from build123d import *

# Parameters (mm, degrees)
SKETCH1_R           = 2.5019
BOSS_EXTRUDE1_DEPTH = 110.9472
SKETCH2_R           = 19.05
BOSS_EXTRUDE2_DEPTH = 1.5875
SKETCH3_R           = 4.0005
BOSS_EXTRUDE3_DEPTH = 20.5994
CUT_EXTRUDE1_DEPTH  = 105.791


with BuildPart() as part:
    # Sketch1 → Boss-Extrude1 (new body)
    with BuildSketch(Plane.XY):
        with BuildLine():
            Line((-34.002396427, 28.194), (18.143803573, 28.194))
            ThreePointArc((18.143803573, 28.194), (19.643506345, 27.572802772), (20.264703573, 26.0731))
            Line((20.264703573, 26.0731), (20.264703573, -26.0731))
            ThreePointArc((20.264703573, -26.0731), (19.643506345, -27.572802772), (18.143803573, -28.194))
            Line((18.143803573, -28.194), (-34.002396427, -28.194))
            ThreePointArc((-34.002396427, -28.194), (-35.502099199, -27.572802772), (-36.123296427, -26.0731))
            Line((-36.123296427, -26.0731), (-36.123296427, 26.0731))
            ThreePointArc((-36.123296427, 26.0731), (-35.502099199, 27.572802772), (-34.002396427, 28.194))
        make_face()
        with Locations((15.641903573, 23.5712)):
            Circle(SKETCH1_R, mode=Mode.SUBTRACT)
        with Locations(Location((-31.500496427, 23.5712, 0), (0, 0, 180))):
            Circle(SKETCH1_R, mode=Mode.SUBTRACT)
        with Locations((-31.500496427, -23.5712)):
            Circle(SKETCH1_R, mode=Mode.SUBTRACT)
        with Locations(Location((15.641903573, -23.5712, 0), (0, 0, 180))):
            Circle(SKETCH1_R, mode=Mode.SUBTRACT)
    extrude(amount=BOSS_EXTRUDE1_DEPTH)

    # Sketch2 → Boss-Extrude2 (add)
    with BuildSketch(Plane.XY.offset(110.9472)):
        with Locations((-7.929296427, 0)):
            Circle(SKETCH2_R)
    extrude(amount=BOSS_EXTRUDE2_DEPTH)

    # Sketch3 → Boss-Extrude3 (add)
    with BuildSketch(Plane.XY.offset(112.5347)):
        with Locations((-7.929296427, 0)):
            Circle(SKETCH3_R)
    extrude(amount=BOSS_EXTRUDE3_DEPTH)

    # Sketch4 → Cut-Extrude1 (cut)
    with BuildSketch(Plane(origin=(0, 0, 0), x_dir=(-1, 0, 0), z_dir=(0, 0, -1))):
        with BuildLine():
            Line((34.535796427, -19.177), (33.456296427, -19.177))
            ThreePointArc((33.456296427, -19.177), (28.966168367, -21.036871939), (27.106296427, -25.527))
            Line((27.106296427, -25.527), (27.106296427, -26.6065))
            ThreePointArc((27.106296427, -26.6065), (26.641328442, -27.729032015), (25.518796427, -28.194))
            Line((25.518796427, -28.194), (18.677208221, -28.194))
            Line((18.677208221, -28.194), (18.677208221, -39.079996732))
            Line((18.677208221, -39.079996732), (53.323924266, -39.079996732))
            Line((53.323924266, -39.079996732), (53.323924266, -7.667262783))
            Line((53.323924266, -7.667262783), (36.123296427, -7.667262783))
            Line((36.123296427, -7.667262783), (36.123296427, -17.5895))
            ThreePointArc((36.123296427, -17.5895), (35.658328442, -18.712032015), (34.535796427, -19.177))
        make_face()
        with BuildLine():
            Line((36.123296427, 7.667262783), (36.123296427, 17.5895))
            ThreePointArc((36.123296427, 17.5895), (35.658328442, 18.712032015), (34.535796427, 19.177))
            Line((34.535796427, 19.177), (33.456296427, 19.177))
            ThreePointArc((33.456296427, 19.177), (28.966168367, 21.036871939), (27.106296427, 25.527))
            Line((27.106296427, 25.527), (27.106296427, 26.6065))
            ThreePointArc((27.106296427, 26.6065), (26.641328442, 27.729032015), (25.518796427, 28.194))
            Line((25.518796427, 28.194), (18.677208221, 28.194))
            Line((18.677208221, 28.194), (18.677208221, 39.079996732))
            Line((18.677208221, 39.079996732), (53.323924266, 39.079996732))
            Line((53.323924266, 39.079996732), (53.323924266, 7.667262783))
            Line((53.323924266, 7.667262783), (36.123296427, 7.667262783))
        make_face()
        with BuildLine():
            Line((-18.677203573, 19.177), (-17.597703573, 19.177))
            ThreePointArc((-17.597703573, 19.177), (-13.107575512, 21.036871939), (-11.247703573, 25.527))
            Line((-11.247703573, 25.527), (-11.247703573, 26.6065))
            ThreePointArc((-11.247703573, 26.6065), (-10.782735588, 27.729032015), (-9.660203573, 28.194))
            Line((-9.660203573, 28.194), (-2.818615366, 28.194))
            Line((-2.818615366, 28.194), (-2.818615366, 39.079996732))
            Line((-2.818615366, 39.079996732), (-37.465331412, 39.079996732))
            Line((-37.465331412, 39.079996732), (-37.465331412, 7.667262783))
            Line((-37.465331412, 7.667262783), (-20.264703573, 7.667262783))
            Line((-20.264703573, 7.667262783), (-20.264703573, 17.5895))
            ThreePointArc((-20.264703573, 17.5895), (-19.799735588, 18.712032015), (-18.677203573, 19.177))
        make_face()
        with BuildLine():
            Line((-20.264703573, -7.667262783), (-20.264703573, -17.5895))
            ThreePointArc((-20.264703573, -17.5895), (-19.799735588, -18.712032015), (-18.677203573, -19.177))
            Line((-18.677203573, -19.177), (-17.597703573, -19.177))
            ThreePointArc((-17.597703573, -19.177), (-13.107575512, -21.036871939), (-11.247703573, -25.527))
            Line((-11.247703573, -25.527), (-11.247703573, -26.6065))
            ThreePointArc((-11.247703573, -26.6065), (-10.782735588, -27.729032015), (-9.660203573, -28.194))
            Line((-9.660203573, -28.194), (-2.818615366, -28.194))
            Line((-2.818615366, -28.194), (-2.818615366, -39.079996732))
            Line((-2.818615366, -39.079996732), (-37.465331412, -39.079996732))
            Line((-37.465331412, -39.079996732), (-37.465331412, -7.667262783))
            Line((-37.465331412, -7.667262783), (-20.264703573, -7.667262783))
        make_face()
    extrude(amount=-CUT_EXTRUDE1_DEPTH, mode=Mode.SUBTRACT)


solid = part.part
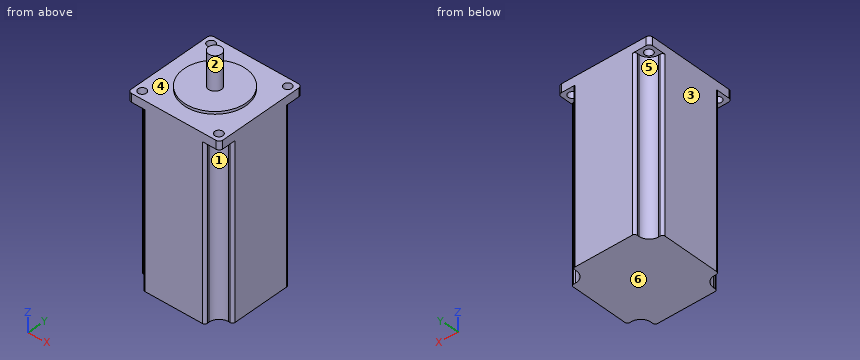
Here's how the part is built. I have some questions about the finished solid (model axes, mm). Face numbers are marked on the shaded views. A direction names the side the tool comes from. Coordinates: 2 decimals unless noted, no trailing zeros. Write each loop counter-clockwise with the first axis right and the second up, starting at its lowest first coordinate (ties: lowest second). Pieces come first, ordered by that corner, then holes. Notation, with made-up numbers: (28, 20.5) - (42, 20.5) arc R17 ccw to (42, 27.5) - close; hole circle Ø11 at (87.25, -10.75). An arc over 180 degrees is marked (long way). Use one line per item in the form item = value.
1) I need wall thicknesses on line 1 (Z direction, x = 12, y = 2.5); line 2 (Z direction, x = -12, y = -16.5); line 3 (X direction, y = -25, z = 6). Which ranges of each line are inside material? Lowest first, please.
Solved:
line_1 = 0 to 110.95
line_2 = 0 to 112.53
line_3 = -27.13 to 11.27
2) Suppose I cut it at D-D, the plane x = -19.5. Write out the boundary of the cut face in (y, z).
Solved:
outline = (-28.19, 0) - (28.19, 0) - (28.19, 110.95) - (15.13, 110.95) - (15.13, 112.53) - (-15.13, 112.53) - (-15.13, 110.95) - (-28.19, 110.95) - close
3) Suppose I cut it at B-B, the plane x = -31.5. Write out the boundary of the cut face in (y, z).
Solved:
outline = (-28.19, 105.79) - (-26.07, 105.79) - (-26.07, 110.95) - (-28.19, 110.95) - close; (-21.07, 105.79) - (-19.49, 105.79) - (-19.49, 0) - (19.49, 0) - (19.49, 105.79) - (21.07, 105.79) - (21.07, 110.95) - (-21.07, 110.95) - close; (26.07, 105.79) - (28.19, 105.79) - (28.19, 110.95) - (26.07, 110.95) - close
4) Suppose I cut it at A-A, the plane y = 0. Write out the boundary of the cut face in (x, z).
Solved:
outline = (-36.12, 0) - (20.26, 0) - (20.26, 110.95) - (11.12, 110.95) - (11.12, 112.53) - (-3.93, 112.53) - (-3.93, 133.13) - (-11.93, 133.13) - (-11.93, 112.53) - (-26.98, 112.53) - (-26.98, 110.95) - (-36.12, 110.95) - close
5) I'm going to push flat-ended pins straight in: P1, Ø1, axis at x = 7.5, y = -22, coming from the +Z side; P2, Ø0.9, axis at y = 26, z = 54, coming from the -X side; P3, Ø1.2, axis at y = -26, z = 76, coming from the +X side. Where does each tip first touch, or does it pass through?
Solved:
P1 = 110.95
P2 = -27.11
P3 = 11.25
6) On a 3-axis mill with a long thin cutter (end or side, diameter ignored), from which of +Z, -Z, +X, -X, +Y, -Y can I reach the whole of each face in a straight line? I mean the marked faces 1, 2 and 3. Say none if no direction works.
Solved:
face_1 = -Z, +X, -Y
face_2 = +Z
face_3 = +Z, -Z, -X, +Y, -Y
7) Thinking about a two-plate mould opening in Z: for the marked faces 4, 5 and 6, which applies, released by +Z, released by -Z, zero draft, split by the parting line, or undercut?
Solved:
face_4 = released by +Z
face_5 = zero draft
face_6 = released by -Z
